from build123d import *

# Parameters (mm, degrees)
F0_W     = 15.59283
F0_H     = 12.481529
F1_DEPTH = 32.004


with BuildPart() as f1:
    # F0 (on Top) → F1 (new body)
    with BuildSketch(Plane.XY):
        Polygon((-16.001523, -7.900454), (20.335106, -7.900454), (20.335106, 20.730838), (10.882463, 20.730838), (-16.001523, 20.730838), align=None)
        Polygon((20.335106, 20.730838), (20.335106, -7.900454), (35.927936, 20.730838), align=None)
        with Locations((28.131521, 26.971602)):
            Rectangle(F0_W, F0_H)
        Polygon((10.882463, 20.730838), (20.335106, 20.730838), (20.335106, 33.212367), (-16.001523, 20.730838), align=None)
    extrude(amount=F1_DEPTH)


solid = f1.part
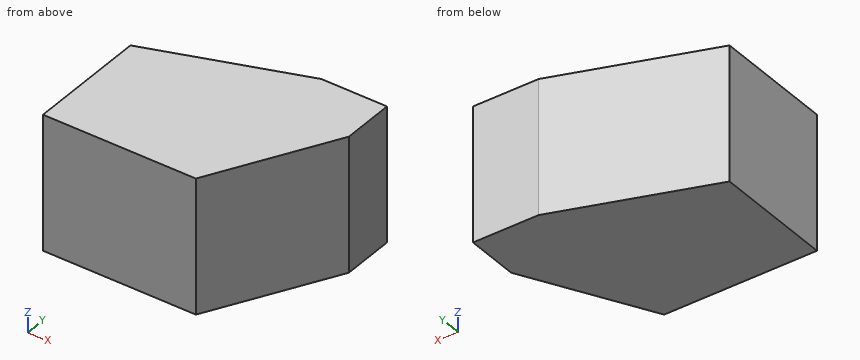
Geometry: final body of the model. Coordinates: model frame, mm. Give positions to 0.01 mm unless a question says otherwise; leave off trailing zeros. Write each loop counter-clockwise with the first axis right and the second up, starting at its lowest first coordinate (ties: lowest second). Pieces come first, ordered by that corner, then holes. Notation, with made-up numbers: M 54,76.5 L 75,76.5 A20 cw 75,91.5 Z; hole C -28,70.25 d7. An arc over 180 degrees is marked long. Answer in a Markdown table with one row per item. Add a question column.
(1) Section B-B on y = 8.5. Return loops of the section in (x, z).
(2) Ray query, line 1 (Y direction, x = 32, z = 12.5); line 2 (Y direction, x = -12.5, z = 27); line 3 (X direction, y = 16, z = 27). Return the intervals inside material, ascending.
(3) Section A-A on z = 3. Return loops of the section in (x, y).
(4) First-contact query: pin 1 (6 mm diameter, centred on y = 16.5, z = 19.5, fed in from +X); pin 2 (5 mm diameter, centred on x = 3.5, z = 13, fed in from +Y). Flat tips, straight axial feed; report the tip coordinate or a pass-through.
(5) Section C-C on x = -8. Return loops of the section in (y, z), and give its area (3 significant figures).
Result set:
| question | item | result |
|---|---|---|
| 1 | outline | M -16,0 L 29.27,0 L 29.27,32 L -16,32 Z |
| 2 | line 1 | y = 13.52 to 33.21 |
| 2 | line 2 | y = -7.9 to 21.93 |
| 2 | line 3 | x = -16 to 33.35 |
| 3 | outline | M -16,-7.9 L 20.34,-7.9 L 35.93,20.73 L 35.93,33.21 L 20.34,33.21 L -16,20.73 Z |
| 4 | pin 1 | stops at x = 35.26 |
| 4 | pin 2 | stops at y = 28.29 |
| 5 | outline | M -7.9,0 L 23.48,0 L 23.48,32 L -7.9,32 Z |
| 5 | area | 1,000 mm^2 |
